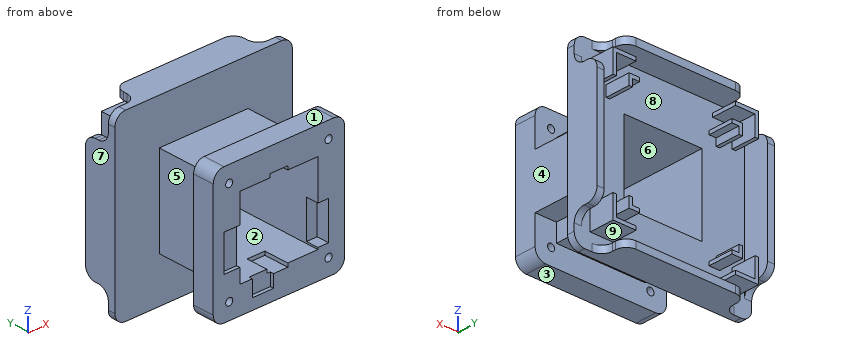
```python
from build123d import *

# Parameters (mm, degrees)
SKETCH_2_W            = 37
SKETCH_2_H            = 37
EXTRUDE_1_DEPTH       = 23
SKETCH_3_W            = 22
SKETCH_3_H            = 22
CUT_EXTRUDE_1_DEPTH   = 23
SKETCH_19_OUTSIDE_W   = 50.432
SKETCH_19_OUTSIDE_H   = 50.432
SKETCH_19_OUTSIDE_W_2 = 25
SKETCH_19_OUTSIDE_H_2 = 25
CUT_EXTRUDE_17_DEPTH  = 17
SKETCH_4_W            = 50
SKETCH_4_H            = 50
EXTRUDE_2_DEPTH       = 9
SKETCH_5_W            = 46
SKETCH_5_H            = 46
CUT_EXTRUDE_3_DEPTH   = 7
SKETCH_12_W           = 8
SKETCH_12_H           = 8
CUT_EXTRUDE_14_DEPTH  = 14
SKETCH_6_W            = 22
SKETCH_6_H            = 22
CUT_EXTRUDE_4_DEPTH   = 2
SKETCH_11_R           = 1
CUT_EXTRUDE_7_DEPTH   = 8
SKETCH_13_W           = 41
SKETCH_13_H           = 41
SKETCH_13_W_2         = 39
SKETCH_13_H_2         = 39
EXTRUDE_3_DEPTH       = 7
SKETCH_17_W           = 32
SKETCH_17_H           = 32
SKETCH_17_W_2         = 30
SKETCH_17_H_2         = 30
EXTRUDE_4_DEPTH       = 7
SKETCH_15_W           = 28
SKETCH_15_H           = 1
SKETCH_15_W_2         = 1
SKETCH_15_H_2         = 28
CUT_EXTRUDE_15_DEPTH  = 7
SKETCH_18_W           = 1
SKETCH_18_H           = 26
SKETCH_18_W_2         = 26
SKETCH_18_H_2         = 1
CUT_EXTRUDE_16_DEPTH  = 7
SKETCH_20_W           = 3
SKETCH_20_H           = 10.5
CUT_EXTRUDE_18_DEPTH  = 3.5
SKETCH_21_W           = 4.5
SKETCH_21_H           = 10
CUT_EXTRUDE_19_DEPTH  = 1
SKETCH_22_W           = 5
SKETCH_22_H           = 1
CUT_EXTRUDE_21_DEPTH  = 7
SKETCH_24_W           = 6
SKETCH_24_H           = 4.5
CUT_EXTRUDE_22_DEPTH  = 1
SKETCH_25_W           = 6
SKETCH_25_H           = 15
EXTRUDE_5_DEPTH       = 17
FILLET_5_R            = 3
FILLET_6_R            = 3
FILLET_10_R           = 3
FILLET_11_R           = 3
FILLET_12_R           = 3
FILLET_14_R           = 3
FILLET_15_R           = 3
FILLET_16_R           = 3
FILLET_19_R           = 3
FILLET_20_R           = 3
FILLET_21_R           = 3
FILLET_22_R           = 3
FILLET_28_R           = 3
FILLET_29_R           = 3
FILLET_30_R           = 3
FILLET_31_R           = 3
FILLET_32_R           = 3
FILLET_33_R           = 3
FILLET_34_R           = 3
FILLET_35_R           = 3
FILLET_36_R           = 3
FILLET_37_R           = 3
FILLET_38_R           = 3
FILLET_39_R           = 3


with BuildPart() as part:
    # 草图2 → 凸台-拉伸1 (new body)
    with BuildSketch(Plane(origin=(0, 0, 0), x_dir=(1, 0, 0), z_dir=(0, 1, 0))):
        Rectangle(SKETCH_2_W, SKETCH_2_H)
    extrude(amount=EXTRUDE_1_DEPTH)

    # 草图3 → 切除-拉伸1 (cut)
    with BuildSketch(Plane.XZ):
        Rectangle(SKETCH_3_W, SKETCH_3_H)
    extrude(amount=-CUT_EXTRUDE_1_DEPTH, mode=Mode.SUBTRACT)

    # 草图19 outside → 切除-拉伸17 (cut)
    with BuildSketch(Plane(origin=(0, 6, 0), x_dir=(-1, 0, 0), z_dir=(0, -1, 0))):
        Rectangle(SKETCH_19_OUTSIDE_W, SKETCH_19_OUTSIDE_H)
        Rectangle(SKETCH_19_OUTSIDE_W_2, SKETCH_19_OUTSIDE_H_2, mode=Mode.SUBTRACT)
    extrude(amount=-CUT_EXTRUDE_17_DEPTH, mode=Mode.SUBTRACT)

    # 草图4 → 凸台-拉伸2 (add)
    with BuildSketch(Plane(origin=(0, 23, 0), x_dir=(1, 0, 0), z_dir=(0, 1, 0))):
        Rectangle(SKETCH_4_W, SKETCH_4_H)
    extrude(amount=EXTRUDE_2_DEPTH)

    # 草图5 → 切除-拉伸3 (cut)
    with BuildSketch(Plane(origin=(0, 32, 0), x_dir=(1, 0, 0), z_dir=(0, 1, 0))):
        Rectangle(SKETCH_5_W, SKETCH_5_H)
    extrude(amount=-CUT_EXTRUDE_3_DEPTH, mode=Mode.SUBTRACT)

    # 草图12 → 切除-拉伸14 (cut)
    with BuildSketch(Plane(origin=(0, 25, 0), x_dir=(1, 0, 0), z_dir=(0, 1, 0))):
        with Locations((-21, -21)):
            Rectangle(SKETCH_12_W, SKETCH_12_H)
        with Locations((-21, 21)):
            Rectangle(SKETCH_12_W, SKETCH_12_H)
        with Locations((21, 21)):
            Rectangle(SKETCH_12_W, SKETCH_12_H)
        with Locations((21, -21)):
            Rectangle(SKETCH_12_W, SKETCH_12_H)
    extrude(amount=CUT_EXTRUDE_14_DEPTH, mode=Mode.SUBTRACT)

    # 草图6 → 切除-拉伸4 (cut)
    with BuildSketch(Plane(origin=(0, 25, 0), x_dir=(1, 0, 0), z_dir=(0, 1, 0))):
        Rectangle(SKETCH_6_W, SKETCH_6_H)
    extrude(amount=-CUT_EXTRUDE_4_DEPTH, mode=Mode.SUBTRACT)

    # 草图11 → 切除-拉伸7 (cut)
    with BuildSketch(Plane.XZ):
        with Locations(Location((14, 14, 0), (0, 0, 270))):
            Circle(SKETCH_11_R)
        with Locations(Location((14, -14, 0), (0, 0, 270))):
            Circle(SKETCH_11_R)
        with Locations(Location((-14, -14, 0), (0, 0, 270))):
            Circle(SKETCH_11_R)
        with Locations(Location((-14, 14, 0), (0, 0, 270))):
            Circle(SKETCH_11_R)
    extrude(amount=-CUT_EXTRUDE_7_DEPTH, mode=Mode.SUBTRACT)

    # 草图13 → 凸台-拉伸3 (add)
    with BuildSketch(Plane(origin=(0, 25, 0), x_dir=(1, 0, 0), z_dir=(0, 1, 0))):
        Rectangle(SKETCH_13_W, SKETCH_13_H)
        Rectangle(SKETCH_13_W_2, SKETCH_13_H_2, mode=Mode.SUBTRACT)
    extrude(amount=EXTRUDE_3_DEPTH)

    # 草图17 → 凸台-拉伸4 (add)
    with BuildSketch(Plane(origin=(0, 25, 0), x_dir=(1, 0, 0), z_dir=(0, 1, 0))):
        Rectangle(SKETCH_17_W, SKETCH_17_H)
        Rectangle(SKETCH_17_W_2, SKETCH_17_H_2, mode=Mode.SUBTRACT)
    extrude(amount=EXTRUDE_4_DEPTH)

    # 草图15 → 切除-拉伸15 (cut)
    with BuildSketch(Plane(origin=(0, 25, 0), x_dir=(1, 0, 0), z_dir=(0, 1, 0))):
        with Locations((0, -20)):
            Rectangle(SKETCH_15_W, SKETCH_15_H)
        with Locations((20, 0)):
            Rectangle(SKETCH_15_W_2, SKETCH_15_H_2)
        with Locations((-20, 0)):
            Rectangle(SKETCH_15_W_2, SKETCH_15_H_2)
        with Locations((0, 20)):
            Rectangle(SKETCH_15_W, SKETCH_15_H)
    extrude(amount=CUT_EXTRUDE_15_DEPTH, mode=Mode.SUBTRACT)

    # 草图18 → 切除-拉伸16 (cut)
    with BuildSketch(Plane(origin=(0, 25, 0), x_dir=(1, 0, 0), z_dir=(0, 1, 0))):
        with Locations((15.5, 0)):
            Rectangle(SKETCH_18_W, SKETCH_18_H)
        with Locations((0, -15.5)):
            Rectangle(SKETCH_18_W_2, SKETCH_18_H_2)
        with Locations((-15.5, 0)):
            Rectangle(SKETCH_18_W, SKETCH_18_H)
        with Locations((0, 15.5)):
            Rectangle(SKETCH_18_W_2, SKETCH_18_H_2)
    extrude(amount=CUT_EXTRUDE_16_DEPTH, mode=Mode.SUBTRACT)

    # 草图20 → 切除-拉伸18 (cut)
    with BuildSketch(Plane.XZ):
        with Locations((12.5, -5.25)):
            Rectangle(SKETCH_20_W, SKETCH_20_H)
    extrude(amount=-CUT_EXTRUDE_18_DEPTH, mode=Mode.SUBTRACT)

    # 草图21 → 切除-拉伸19 (cut)
    with BuildSketch(Plane.XZ):
        with Locations((-13.25, -2)):
            Rectangle(SKETCH_21_W, SKETCH_21_H)
    extrude(amount=-CUT_EXTRUDE_19_DEPTH, mode=Mode.SUBTRACT)

    # 草图22 → 切除-拉伸21 (cut)
    with BuildSketch(Plane.XZ):
        with Locations((0, -11.5)):
            Rectangle(SKETCH_22_W, SKETCH_22_H)
        with Locations((0, 11.5)):
            Rectangle(SKETCH_22_W, SKETCH_22_H)
    extrude(amount=-CUT_EXTRUDE_21_DEPTH, mode=Mode.SUBTRACT)

    # 草图24 → 切除-拉伸22 (cut)
    with BuildSketch(Plane.XZ):
        with Locations((-4.5, -13.25)):
            Rectangle(SKETCH_24_W, SKETCH_24_H)
    extrude(amount=-CUT_EXTRUDE_22_DEPTH, mode=Mode.SUBTRACT)

    # 草图25 → 凸台-拉伸5 (add)
    with BuildSketch(Plane(origin=(0, 6, 0), x_dir=(1, 0, 0), z_dir=(0, 1, 0))):
        with Locations((15.5, 0)):
            Rectangle(SKETCH_25_W, SKETCH_25_H)
    extrude(amount=EXTRUDE_5_DEPTH)

    # 圆角5
    fillet_5_edges = [part.edges().sort_by_distance(p)[0] for p in [
        (25, 24, -25),
    ]]
    fillet(fillet_5_edges, radius=FILLET_5_R)

    # 圆角6
    fillet_6_edges = [part.edges().sort_by_distance(p)[0] for p in [
        (25, 24, 25),
    ]]
    fillet(fillet_6_edges, radius=FILLET_6_R)

    # 圆角10
    fillet_10_edges = [part.edges().sort_by_distance(p)[0] for p in [
        (17, 25, -24),
    ]]
    fillet(fillet_10_edges, radius=FILLET_10_R)

    # 圆角11
    fillet_11_edges = [part.edges().sort_by_distance(p)[0] for p in [
        (24, 32, -17),
    ]]
    fillet(fillet_11_edges, radius=FILLET_11_R)

    # 圆角12
    fillet_12_edges = [part.edges().sort_by_distance(p)[0] for p in [
        (24, 25, -17),
    ]]
    fillet(fillet_12_edges, radius=FILLET_12_R)

    # 圆角14
    fillet_14_edges = [part.edges().sort_by_distance(p)[0] for p in [
        (17, 25, 24),
    ]]
    fillet(fillet_14_edges, radius=FILLET_14_R)

    # 圆角15
    fillet_15_edges = [part.edges().sort_by_distance(p)[0] for p in [
        (24, 32, 17),
    ]]
    fillet(fillet_15_edges, radius=FILLET_15_R)

    # 圆角16
    fillet_16_edges = [part.edges().sort_by_distance(p)[0] for p in [
        (24, 25, 17),
    ]]
    fillet(fillet_16_edges, radius=FILLET_16_R)

    # 圆角19
    fillet_19_edges = [part.edges().sort_by_distance(p)[0] for p in [
        (-18.5, 3, -18.5),
    ]]
    fillet(fillet_19_edges, radius=FILLET_19_R)

    # 圆角20
    fillet_20_edges = [part.edges().sort_by_distance(p)[0] for p in [
        (-18.5, 3, 18.5),
    ]]
    fillet(fillet_20_edges, radius=FILLET_20_R)

    # 圆角21
    fillet_21_edges = [part.edges().sort_by_distance(p)[0] for p in [
        (18.5, 3, 18.5),
    ]]
    fillet(fillet_21_edges, radius=FILLET_21_R)

    # 圆角22
    fillet_22_edges = [part.edges().sort_by_distance(p)[0] for p in [
        (18.5, 3, -18.5),
    ]]
    fillet(fillet_22_edges, radius=FILLET_22_R)

    # 圆角28
    fillet_28_edges = [part.edges().sort_by_distance(p)[0] for p in [
        (-17, 25, -24),
    ]]
    fillet(fillet_28_edges, radius=FILLET_28_R)

    # 圆角29
    fillet_29_edges = [part.edges().sort_by_distance(p)[0] for p in [
        (-24, 25, -17),
    ]]
    fillet(fillet_29_edges, radius=FILLET_29_R)

    # 圆角30
    fillet_30_edges = [part.edges().sort_by_distance(p)[0] for p in [
        (-24, 25, 17),
    ]]
    fillet(fillet_30_edges, radius=FILLET_30_R)

    # 圆角31
    fillet_31_edges = [part.edges().sort_by_distance(p)[0] for p in [
        (-17, 25, 24),
    ]]
    fillet(fillet_31_edges, radius=FILLET_31_R)

    # 圆角32
    fillet_32_edges = [part.edges().sort_by_distance(p)[0] for p in [
        (17, 32, 24),
    ]]
    fillet(fillet_32_edges, radius=FILLET_32_R)

    # 圆角33
    fillet_33_edges = [part.edges().sort_by_distance(p)[0] for p in [
        (-17, 32, 24),
    ]]
    fillet(fillet_33_edges, radius=FILLET_33_R)

    # 圆角34
    fillet_34_edges = [part.edges().sort_by_distance(p)[0] for p in [
        (17, 32, -24),
    ]]
    fillet(fillet_34_edges, radius=FILLET_34_R)

    # 圆角35
    fillet_35_edges = [part.edges().sort_by_distance(p)[0] for p in [
        (-17, 32, -24),
    ]]
    fillet(fillet_35_edges, radius=FILLET_35_R)

    # 圆角36
    fillet_36_edges = [part.edges().sort_by_distance(p)[0] for p in [
        (-24, 32, 17),
    ]]
    fillet(fillet_36_edges, radius=FILLET_36_R)

    # 圆角37
    fillet_37_edges = [part.edges().sort_by_distance(p)[0] for p in [
        (-24, 32, -17),
    ]]
    fillet(fillet_37_edges, radius=FILLET_37_R)

    # 圆角38
    fillet_38_edges = [part.edges().sort_by_distance(p)[0] for p in [
        (-25, 24, 25),
    ]]
    fillet(fillet_38_edges, radius=FILLET_38_R)

    # 圆角39
    fillet_39_edges = [part.edges().sort_by_distance(p)[0] for p in [
        (-25, 24, -25),
    ]]
    fillet(fillet_39_edges, radius=FILLET_39_R)


solid = part.part
```
Build history of the part. All positions in model axes, mm. Face numbers are marked on the shaded views. A direction names the side the tool comes from. Give positions to 0.01 mm unless a question says otherwise; leave off trailing zeros. Loops run counter-clockwise (first coordinate to the right, second up) from the corner with the lowest first, then second, coordinate; pieces in that order, holes last. Notation, with made-up numbers: (30, -14.75) -> (79, -14.75) arc R7 cw to (79, -2.75) -> close; hole circle Ø4 at (48, -22). An arc over 180 degrees is marked (long way). One line per question, with ' | ' between items. Start each with the question number.
1) Probe L1, parallel to X at y = 1.2, z = 14; L2, parallel to Z at x = 1, y = 27.5; L3, parallel to Z at x = -3, y = 8.5. List the from-to ranges inside material, lowest first.
2) Two-plate mould, pull along X, no slides. Class the marked faces 6, 7, 8 and 9: released by +X, released by -X, zero draft, split by the parting line, or undercut.
3) 3-axis set-ups, long thin cutter, end or side, ignore diameter. For the marked faces 1, 2, 3, 4 and 5: which of +Z, -Z, +X, -X, +Y, -Y reach the whole face in a straight line?
4) Cut at C-C (x = 6). Give the cut face in (y, z), plus the area to 3 significant figures.
5) Cut at D-D (z = 1). Give the cut face in (x, y).
6) Cut at B-B (z = -6). Give the cut face in (x, y), plus the area to 3 significant figures.
7) Pin check, flat tips, straight feed: pin 1 (5 mm diameter, centred on x = 5, y = 14, fed in from +Z); pin 2 (3 mm diameter, centred on x = 12, y = 12, fed in from -Z); pin 3 (1.1 mm diameter, centred on y = 28.5, z = -24, fed in from +X). Stop position of each tip, or through.
8) Cut at A-A (y = 10). Give the cut face in (x, z).
Return value:
1) L1: -18.5 to -15, -13 to 13, 15 to 18.5 | L2: -25 to -23, 23 to 25 | L3: -12.5 to -11, 11 to 12.5
2) face 6: undercut | face 7: released by -X | face 8: undercut | face 9: zero draft
3) face 1: +Z, +X, -X, -Y | face 2: +Y, -Y | face 3: -Z, +X, -X, -Y | face 4: +Z, -Z, +X, -Y | face 5: +Z, -Z, -X
4) outline: (0, -18.5) -> (6, -18.5) -> (6, -12.5) -> (23, -12.5) -> (23, -25) -> (32, -25) -> (32, -23) -> (25, -23) -> (25, -11) -> (0, -11) -> close; (0, 11) -> (25, 11) -> (25, 23) -> (32, 23) -> (32, 25) -> (23, 25) -> (23, 12.5) -> (6, 12.5) -> (6, 18.5) -> (0, 18.5) -> close | area: 225 mm^2
5) outline: (-25, 23) -> (-12.5, 23) -> (-12.5, 6) -> (-18.5, 6) -> (-18.5, 0) -> (-15.5, 0) -> (-15.5, 1) -> (-11, 1) -> (-11, 25) -> (-23, 25) -> (-23, 32) -> (-25, 32) -> close; (11, 0) -> (18.5, 0) -> (18.5, 23) -> (25, 23) -> (25, 32) -> (23, 32) -> (23, 25) -> (11, 25) -> close
6) outline: (-25, 23) -> (-12.5, 23) -> (-12.5, 6) -> (-18.5, 6) -> (-18.5, 0) -> (-15.5, 0) -> (-15.5, 1) -> (-11, 1) -> (-11, 25) -> (-23, 25) -> (-23, 32) -> (-25, 32) -> close; (11, 3.5) -> (14, 3.5) -> (14, 0) -> (18.5, 0) -> (18.5, 23) -> (25, 23) -> (25, 32) -> (23, 32) -> (23, 25) -> (11, 25) -> close | area: 312 mm^2
7) pin 1: z = 12.5 | pin 2: z = -12.5 | pin 3: x = 17
8) outline: (-12.5, -12.5) -> (12.5, -12.5) -> (12.5, -7.5) -> (18.5, -7.5) -> (18.5, 7.5) -> (12.5, 7.5) -> (12.5, 12.5) -> (-12.5, 12.5) -> close; hole (-11, -11) -> (11, -11) -> (11, 11) -> (-11, 11) -> close
